Can you work these out from the model? Positions are in its coordinate system, mm. Face numbers are marked on the shaded views. Coordinates: 2 decimals unless noted, no trailing zeros. Write each loop counter-clockwise with the first axis right and the second up, starting at its lowest first coordinate (ties: lowest second). Pieces come first, ordered by that corner, then holes.
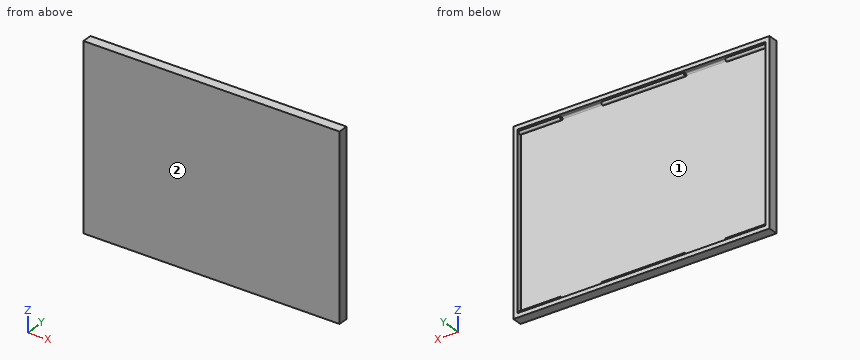
```python
from build123d import *

# Parameters (mm, degrees)
SKETCH_1_W          = 310
SKETCH_1_H          = 220
EXTRUDE_1_DEPTH     = 12
SKETCH_2_W          = 300
SKETCH_2_H          = 210
CUT_EXTRUDE_4_DEPTH = 6
SKETCH_6_W          = 300
SKETCH_6_H          = 2
EXTRUDE_3_DEPTH     = 2
SKETCH_8_R          = 2
CUT_EXTRUDE_5_DEPTH = 300
SKETCH_8_2_R        = 2
SKETCH_8_2_R_2      = 1.5
EXTRUDE_1_2_DEPTH   = 300
SKETCH_10_R         = 2
CUT_EXTRUDE_6_DEPTH = 300
SKETCH_10_2_R       = 2
SKETCH_10_2_R_2     = 1.5
EXTRUDE_2_DEPTH     = 300
SKETCH_12_R         = 2
CUT_EXTRUDE_7_DEPTH = 50
SKETCH_13_R         = 2
CUT_EXTRUDE_8_DEPTH = 50


with BuildPart() as part:
    # 草图1 → Extrude 1 (new body)
    with BuildSketch(Plane(origin=(0, 0, 0), x_dir=(1, 0, 0), z_dir=(0, 1, 0))):
        with Locations((0.660377358, 22.830188679)):
            Rectangle(SKETCH_1_W, SKETCH_1_H)
    extrude(amount=EXTRUDE_1_DEPTH)

    # 草图2 → 切除-拉伸4 (cut)
    with BuildSketch(Plane(origin=(0, 12, 0), x_dir=(1, 0, 0), z_dir=(0, 1, 0))):
        with Locations((0.660377358, 22.830188679)):
            Rectangle(SKETCH_2_W, SKETCH_2_H)
    extrude(amount=-CUT_EXTRUDE_4_DEPTH, mode=Mode.SUBTRACT)

    # 草图6 → 凸台-拉伸3 (add)
    with BuildSketch(Plane(origin=(0, 6, 0), x_dir=(1, 0, 0), z_dir=(0, 1, 0))):
        with Locations((0.660377358, 126.830188679)):
            Rectangle(SKETCH_6_W, SKETCH_6_H)
        with Locations((0.660377358, -81.169811321)):
            Rectangle(SKETCH_6_W, SKETCH_6_H)
    extrude(amount=EXTRUDE_3_DEPTH)

    # 草图8 → 切除-拉伸5 (cut)
    with BuildSketch(Plane(origin=(150.660377358, 0, 0), x_dir=(0, 0, -1), z_dir=(1, 0, 0))):
        with Locations((-80.169811321, 8)):
            Circle(SKETCH_8_R)
    extrude(amount=-CUT_EXTRUDE_5_DEPTH, mode=Mode.SUBTRACT)

    # 草图8<2> → Extrude 1 2 (add)
    with BuildSketch(Plane(origin=(150.660377358, 0, 0), x_dir=(0, 0, -1), z_dir=(1, 0, 0))):
        with Locations((-80.169811321, 8)):
            Circle(SKETCH_8_2_R)
        with Locations((-80.169811321, 8)):
            Circle(SKETCH_8_2_R_2, mode=Mode.SUBTRACT)
    extrude(amount=-EXTRUDE_1_2_DEPTH)

    # 草图10 → 切除-拉伸6 (cut)
    with BuildSketch(Plane(origin=(150.660377358, 0, 0), x_dir=(0, 0, -1), z_dir=(1, 0, 0))):
        with Locations((125.830188679, 8)):
            Circle(SKETCH_10_R)
    extrude(amount=-CUT_EXTRUDE_6_DEPTH, mode=Mode.SUBTRACT)

    # 草图10<2> → 拉伸-薄壁2 (add)
    with BuildSketch(Plane(origin=(150.660377358, 0, 0), x_dir=(0, 0, -1), z_dir=(1, 0, 0))):
        with Locations((125.830188679, 8)):
            Circle(SKETCH_10_2_R)
        with Locations((125.830188679, 8)):
            Circle(SKETCH_10_2_R_2, mode=Mode.SUBTRACT)
    extrude(amount=-EXTRUDE_2_DEPTH)

    # 草图12 → 切除-拉伸7 (cut)
    with BuildSketch(Plane(origin=(100.660377358, 0, 0), x_dir=(0, 0, -1), z_dir=(1, 0, 0))):
        with Locations((-80.169811321, 8)):
            Circle(SKETCH_12_R)
        with Locations((125.830188679, 8)):
            Circle(SKETCH_12_R)
    extrude(amount=-CUT_EXTRUDE_7_DEPTH, mode=Mode.SUBTRACT)

    # 草图13 → 切除-拉伸8 (cut)
    with BuildSketch(Plane(origin=(-49.339622642, 0, 0), x_dir=(0, 0, -1), z_dir=(1, 0, 0))):
        with Locations((-80.169811321, 8)):
            Circle(SKETCH_13_R)
        with Locations((125.830188679, 8)):
            Circle(SKETCH_13_R)
    extrude(amount=-CUT_EXTRUDE_8_DEPTH, mode=Mode.SUBTRACT)


solid = part.part
```
1. We'd pull the mould along X, two halves only. Please class the marked faces 1 and 2: released by +X, released by -X, zero draft, split by the parting line, or undercut.
2. I'm going to push flat-ended pins straight in: P1, Ø12, axis at x = 123, z = -25, coming from the -Y side; P2, Ø5, axis at x = -75.5, z = -64, coming from the +Y side. Where does each tip first touch, or does it pass through?
3. If I drill on L1, parallel to X at y = 11.25, z = -80.5; L2, parallel to Z at x = 45.5, y = 7; L3, parallel to Z at x = 37, y = 9.75, over which ranges is the centre line in solid material (lowest first)?
4. If we section it at B-B, the plane z = 56: List the corners of the cut face in (x, y) for me.
5. If we section it at A-A, the plane x = -37.5: List the corners of the cut face in (y, z) for me.
Answers:
1. face 1: undercut
1. face 2: zero draft
2. P1: stops at y = 0
2. P2: stops at y = 6
3. L1: x = -154.34 to -149.34, 150.66 to 155.66
3. L2: z = -132.83 to -126.95, -124.71 to -124.1, 78.44 to 79.05, 81.29 to 87.17
3. L3: z = -132.83 to -127.83, -126.8 to -124.86, 79.2 to 81.14, 82.17 to 87.17
4. outline: (-154.34, 0) - (155.66, 0) - (155.66, 12) - (150.66, 12) - (150.66, 6) - (-149.34, 6) - (-149.34, 12) - (-154.34, 12) - close
5. outline: (0, -132.83) - (12, -132.83) - (12, -127.83) - (8, -127.83) arc R2 ccw (long way) to (6, -125.83) - (6, 80.17) arc R2 ccw (long way) to (8, 82.17) - (12, 82.17) - (12, 87.17) - (0, 87.17) - close; hole circle Ø3 at (8, -125.83); hole circle Ø3 at (8, 80.17)
